Source: CAD feature listing. Evaluate the final solid. Frame: model axes, mm. A direction names the side the tool comes from. Give positions to 0.01 mm unless a question says otherwise; leave off trailing zeros. Write each loop counter-clockwise with the first axis right and the second up, starting at its lowest first coordinate (ties: lowest second). Pieces come first, ordered by that corner, then holes. Notation, with made-up numbers: (28, 68.25) - (64, 68.25) arc R16 ccw to (64, 83.25) - close; hole circle Ø11 at (20.25, 52.25). An arc over 180 degrees is marked (long way). One line per question, with ' | ' between items. Start each with the question number.
(1) Section C-C, the plane y = 34. Return loops of the section in (x, z).
(2) Section A-A, the plane y = 23. Return loops of the section in (x, z).
(3) Draft query along X for faces 1 (the flat face through (0, 3, 9.25)), 2 (the flat face through (20, 22, -4.25)), 3 (the flat face through (-22.5, 2, 0)). Return one class per face: +X half, -X half, draft (parallel to the pull), parting line (faces both ways), or undercut.
(4) Ray query, line 1 (Y direction, x = -20.5, z = -2.25); line 2 (X direction, y = 9, z = -5); line 3 (Z direction, x = 18.5, y = 29.5). Return the intervals inside material, ascending. Write a range as [from, to].
(5) Pin query (flat end, axial travel): pin 1 (6 mm diameter, centred on y = 10.5, z = -4, fed in from -X); pin 2 (5 mm diameter, centred on x = 6, z = 9.5, fed in from -Y); pin 3 (1.5 mm diameter, centred on x = -9.5, z = -1, fed in from +Y). Return the tip coordinate at first contact, or that it passes through.
(6) Section D-D, the plane x = -14.5. Return loops of the section in (y, z), plus the area to 3 significant figures.
(7) Access query for faces 4 (the cylindrical face through (-2.98, 4.57, -12.05)), 5 (the cylindrical face through (11, 3, -7)), 6 (the flat face through (-3, 5, 0)), 7 (the cylindrical face through (17.93, 26.02, 12.05)), 8 (the flat face through (20, 22, 4.25)). Directions: +Z, -Z, +X, -X, +Y, -Y. A direction counts if a zero-diameter tool reaches every point of the face in a straight line with its end or side. Return the directions, or none.
(8) Section B-B, the plane z = 7. Return loops of the section in (x, y).
```python
from build123d import *

# Parameters (mm, degrees)
SKETCH2_W           = 45
SKETCH2_H           = 25
BOSS_EXTRUDE1_DEPTH = 5
CUT_EXTRUDE1_DEPTH  = 27.220221204
SKETCH5_W           = 5
SKETCH5_H           = 25
BOSS_EXTRUDE2_DEPTH = 40
CUT_EXTRUDE2_DEPTH  = 62.491869381
FILLET2_R           = 1.5


with BuildPart() as part:
    # Sketch2 → Boss-Extrude1 (new body)
    with BuildSketch(Plane(origin=(0, 0, 0), x_dir=(1, 0, 0), z_dir=(0, 1, 0))):
        Rectangle(SKETCH2_W, SKETCH2_H)
    extrude(amount=BOSS_EXTRUDE1_DEPTH)

    # Sketch3 → Cut-Extrude1 (cut, through all)
    with BuildSketch(Plane(origin=(0, 5, 0), x_dir=(1, 0, 0), z_dir=(0, 1, 0))):
        with BuildLine():
            Line((-8.75, 9.25), (8.75, 9.25))
            ThreePointArc((8.75, 9.25), (11, 7), (8.75, 4.75))
            Line((8.75, 4.75), (-8.75, 4.75))
            ThreePointArc((-8.75, 4.75), (-11, 7), (-8.75, 9.25))
        make_face()
        with BuildLine():
            Line((-8.75, -4.75), (8.75, -4.75))
            ThreePointArc((8.75, -4.75), (11, -7), (8.75, -9.25))
            Line((8.75, -9.25), (-8.75, -9.25))
            ThreePointArc((-8.75, -9.25), (-11, -7), (-8.75, -4.75))
        make_face()
    extrude(amount=-CUT_EXTRUDE1_DEPTH, mode=Mode.SUBTRACT)

    # Sketch5 → Boss-Extrude2 (add)
    with BuildSketch(Plane(origin=(0, 5, 0), x_dir=(1, 0, 0), z_dir=(0, 1, 0))):
        with Locations((20, 0)):
            Rectangle(SKETCH5_W, SKETCH5_H)
    extrude(amount=BOSS_EXTRUDE2_DEPTH)

    # Sketch6 → Cut-Extrude2 (cut, through all)
    with BuildSketch(Plane.ZY.offset(-17.5)):
        with BuildLine():
            Line((-4.25, 30.25), (-4.25, 13.75))
            ThreePointArc((-4.25, 13.75), (-6, 12), (-7.75, 13.75))
            Line((-7.75, 13.75), (-7.75, 30.25))
            ThreePointArc((-7.75, 30.25), (-6, 32), (-4.25, 30.25))
        make_face()
        with BuildLine():
            Line((7.75, 30.25), (7.75, 13.75))
            ThreePointArc((7.75, 13.75), (6, 12), (4.25, 13.75))
            Line((4.25, 13.75), (4.25, 30.25))
            ThreePointArc((4.25, 30.25), (6, 32), (7.75, 30.25))
        make_face()
    extrude(amount=-CUT_EXTRUDE2_DEPTH, mode=Mode.SUBTRACT)

    # Fillet2
    fillet2_edges = [part.edges().sort_by_distance(p)[0] for p in [
        (-22.5, 5, 0),
        (-2.5, 5, 12.5),
        (-2.5, 5, -12.5),
        (17.5, 5, 0),
        (17.5, 25, -12.5),
        (17.5, 25, 12.5),
        (22.5, 45, 0),
        (22.5, 22.5, 12.5),
        (22.5, 22.5, -12.5),
    ]]
    fillet(fillet2_edges, radius=FILLET2_R)


solid = part.part
```
Check sheet entries:
1) outline: (17.5, -11) arc R1.5 ccw to (19, -12.5) - (21, -12.5) arc R1.5 ccw to (22.5, -11) - (22.5, 11) arc R1.5 ccw to (21, 12.5) - (19, 12.5) arc R1.5 ccw to (17.5, 11) - close
2) outline: (17.5, -11) arc R1.5 ccw to (19, -12.5) - (21, -12.5) arc R1.5 ccw to (22.5, -11) - (22.5, -7.75) - (17.5, -7.75) - close; (17.5, -4.25) - (22.5, -4.25) - (22.5, 4.25) - (17.5, 4.25) - close; (17.5, 7.75) - (22.5, 7.75) - (22.5, 11) arc R1.5 ccw to (21, 12.5) - (19, 12.5) arc R1.5 ccw to (17.5, 11) - close
3) face 1: undercut | face 2: draft | face 3: -X half
4) line 1: [0, 5] | line 2: [17.5, 22.5] | line 3: [-12.41, -7.75], [-4.25, 4.25], [7.75, 12.41]
5) pin 1: x = 17.5 | pin 2: y = 0 | pin 3: y = 5
6) outline: (0, -12.5) - (3.5, -12.5) arc R1.5 ccw to (5, -11) - (5, 11) arc R1.5 ccw to (3.5, 12.5) - (0, 12.5) - close | area: 124 mm²
7) face 4: -Z, -X, +Y | face 5: +Y, -Y | face 6: +Z, -Z, -X, +Y | face 7: +Z, -X, +Y | face 8: +X, -X
8) outline: (-22.5, 0) - (-11, 0) - (-11, 5) - (-21, 5) arc R1.5 ccw to (-22.5, 3.5) - close; (11, 0) - (22.5, 0) - (22.5, 12.31) - (17.5, 12.31) - (17.5, 6.5) arc R1.5 cw to (16, 5) - (11, 5) - close; (17.5, 31.69) - (22.5, 31.69) - (22.5, 43.5) arc R1.5 ccw to (21, 45) - (17.5, 45) - close
